Geometry: see drawing. Coordinates: mm, zero at the bounding-box minimum. Give positions to 0.01 mm unless a question says otherwise; leave off trailing zeros. Write each loop counter-clockwise with the first axis right and the second up, starting at its lowest first coordinate (ties: lowest second). Pieces come first, ordered by that corner, then holes. Notation, with made-up numbers: (78.5, -34) - (94.5, -34) arc R21 cw to (94.5, -27) - close; hole circle Ø8 at (56, -28). An arc over 180 degrees is marked (long way). Answer as CSV lines item,"result". Start each with the question number.
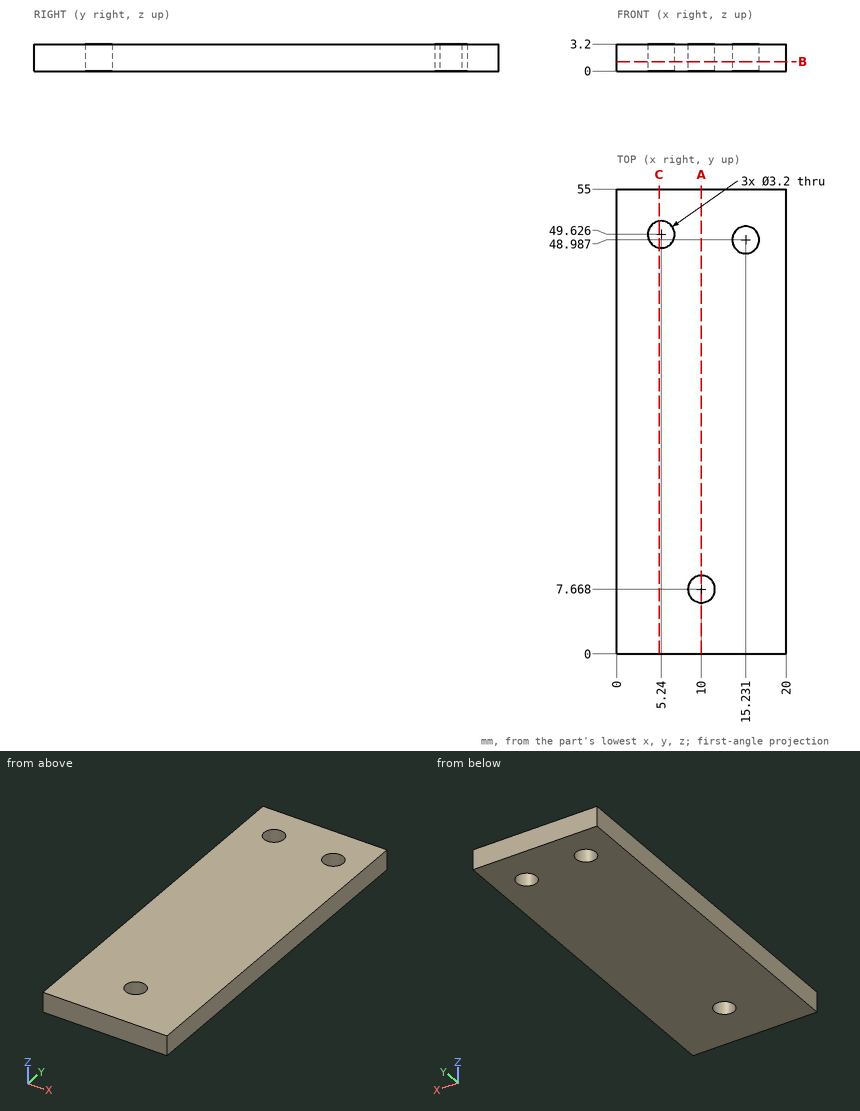
1) Cut plane C-C on x = 5. Output: boundary loops of the cut face in (y, z) (1 decimal), and give its area (3 significant figures).
2) Cut plane A-A on x = 10. Output: boundary loops of the cut face in (y, z).
3) Cut plane B-B on z = 1.1. Output: boundary loops of the cut face in (x, y), and give its area (3 significant figures).
4) Material intervals for line 1 (X direction, y = 49, z = 0.5); line 2 (X direction, y = 50, z = 2.2) (1 decimal); line 3 (X direction, y = 8.5, z = 2.45) (1 decimal), sorted ascending. Write a range as from..to.
5) Contact query for a flat-ended pin moving along its axis: P1, Ø2.5, axis at x = 10, y = 7.67, coming from the +Z side. Output: stop coordinate, or through.
Numbers:
1,outline,"(0, 0) - (48, 0) - (48, 3.2) - (0, 3.2) - close; (51.2, 0) - (55, 0) - (55, 3.2) - (51.2, 3.2) - close"
1,area,"166 mm²"
2,outline,"(0, 0) - (6.07, 0) - (6.07, 3.2) - (0, 3.2) - close; (9.27, 0) - (55, 0) - (55, 3.2) - (9.27, 3.2) - close"
3,outline,"(0, 0) - (20, 0) - (20, 55) - (0, 55) - close; hole circle Ø3.2 at (5.24, 49.63); hole circle Ø3.2 at (10, 7.67); hole circle Ø3.2 at (15.23, 48.99)"
3,area,"1,080 mm²"
4,line 1,"x = 0..3.77, 6.71..13.63, 16.83..20"
4,line 2,"x = 0..3.7, 6.8..14, 16.5..20"
4,line 3,"x = 0..8.6, 11.4..20"
5,P1,"passes through"
